Autodesk Inventor part; units mm, degrees
ref_plane "YZ Plane" through (0, 0, 0) normal (1, 0, 0) x (0, 1, 0)
ref_plane "XZ Plane" through (0, 0, 0) normal (0, 1, 0) x (-1, 0, 0)
ref_plane "XY Plane" through (0, 0, 0) normal (0, 0, 1) x (1, 0, 0)
sketch "Boceto1" plane through (0, 0, 0) normal (0, 1, 0) x (-1, 0, 0)
  line L0 (0, 0) -> (220.8, 0)
  line L1 (220.8, 0) -> (220.8, -220.8)
  line L2 (220.8, -220.8) -> (0, -220.8)
  line L3 (0, -220.8) -> (0, 0)
  line L4 (211.6, -211.6) -> (211.6, -147.2)
  line L5 (211.6, -9.2) -> (156.4, -9.2)
  line L6 (9.2, -211.6) -> (73.6, -211.6)
  line L7 (73.6, -211.6) -> (73.6, -209.3)
  line L8 (75.9, -71.3) -> (211.6, -71.3)
  line L9 (149.5, -211.6) -> (149.5, -75.9)
  line L10 (211.6, -9.2) -> (211.6, -71.3)
  line L11 (211.6, -75.9) -> (211.6, -82.8)
  line L12 (211.6, -211.6) -> (211.6, -75.9)
  line L13 (211.6, -71.3) -> (211.6, -9.2)
  line L14 (75.9, -75.9) -> (144.9, -75.9)
  line L15 (149.5, -75.9) -> (211.6, -75.9)
  line L16 (9.2, -149.5) -> (144.9, -149.5)
  line L17 (144.9, -211.6) -> (144.9, -149.5)
  line L18 (144.9, -144.9) -> (144.9, -75.9)
  line L19 (71.3, -144.9) -> (71.3, -9.2)
  line L20 (9.2, -144.9) -> (71.3, -144.9)
  line L21 (75.9, -144.9) -> (144.9, -144.9)
  line L22 (75.9, -144.9) -> (75.9, -75.9)
  line L23 (75.9, -71.3) -> (75.9, -9.2)
  line L24 (211.6, -9.2) -> (75.9, -9.2)
  line L25 (71.3, -9.2) -> (9.2, -9.2)
  line L26 (9.2, -9.2) -> (9.2, -144.9)
  line L27 (9.2, -149.5) -> (9.2, -211.6)
  line L28 (9.2, -211.6) -> (144.9, -211.6)
  line L29 (149.5, -211.6) -> (211.6, -211.6)
  dimension "d0" = 220.8
  dimension "d1" = 220.8
extrude "Extrusión1" add sketch "Boceto1" along normal blind 4
chamfer "Chaflán1" distance 4 angle 45 4 edges at (-220.8, 4, -110.4) (-110.4, 4, 0) (0, 4, -110.4) (-110.4, 4, -220.8) measured on face at (-121.9, 4, -217.7333)
properties part number "Lampara2"
Part model, mm, in its own coordinate system. Give positions to 0.01 mm unless a question says otherwise; leave off trailing zeros. Use one line per item in the form item = value.
Item 1: Slice it at A-A on z = -124. Count the separate pieces of the cut face and the enclosed holes in it, and give its area (3 significant figures).
Solution:
separate_pieces = 4
enclosed_holes = 0
area = 94.4 mm2
Item 2: Pin check, flat tips, straight feed: pin 1 Ø2 at (x, y) = (-56.5, 2) entering from -Z; pin 2 Ø1.2 at (y, z) = (2.5, -171) entering from -X; pin 3 Ø1.2 at (x, y) = (-160, 2.5) entering from +Z. Stop position of each tip, or through.
Solution:
pin_1 = -219.8
pin_2 = -218.9
pin_3 = -1.9
Item 3: Probe probe 1 along Z at (x, y) = (-172.5, 1.05); probe 2 along X at (y, z) = (3.05, -77); probe 3 along Z at (x, y) = (-113, 1.4). List the from-to ranges inside material, lowest first. Write a range as from..to.
Solution:
probe_1 = -219.75..-211.6, -75.9..-71.3, -9.2..-1.05
probe_2 = -217.75..-211.6, -149.5..-144.9, -75.9..-71.3, -9.2..-3.05
probe_3 = -219.4..-211.6, -149.5..-144.9, -75.9..-71.3, -9.2..-1.4
